For this review, take the finished solid that the model builds, in its own axes (mm). Face numbers are marked on the shaded views. A direction names the side the tool comes from. Round coordinates to 2 decimals unless told otherwise and drop trailing zeros. Write each loop counter-clockwise with the first axis right and the second up, starting at its lowest first coordinate (ties: lowest second). Pieces come first, ordered by that corner, then holes. Notation, with made-up numbers: (67.5, 27.5) - (79.5, 27.5) arc R26 ccw to (79.5, 48.5) - close; hole circle Ø8 at (-11.5, -1). An arc over 180 degrees is marked (long way). One line per item, written item: value. Start each with the question number.
Q1. Add section D-D on z = -15. Write out the cut boundary in (x, y), and give its area (3 significant figures).
Q2. For probe 1 along Z at (x, y) = (-15, 9); probe 2 along X at (y, z) = (9.35, 5); probe 3 along Z at (x, y) = (-15, 1.55), list the stretches that pass through material, from the lowest coordinate up.
Q3. Clearance check with flat-ended pins moving along their axes: pin 1 Ø4 at (y, z) = (19, 5) entering from +X; pin 2 Ø4 at (y, z) = (19.5, 6.5) entering from -X; pin 3 Ø10 at (x, y) = (-26.5, 8) entering from +Z; pin 4 Ø4.5 at (x, z) = (-15, 5) entering from -Y. State where each tip first meets the part, or that it passes through.
Q4. Tool access review of the marked faces 1 and 2: name each direction out of +Z, -Z, +X, -X, +Y, -Y from which nothing blocks a thin tool from reaching the whole face with its end or side.
Q5. Add section A-A on z = 5. Write out the cut boundary in (x, y), and give its area (3 significant figures).
Q6. Add section B-B on x = -15. Write out the cut boundary in (y, z), and give its area (4 significant figures).
Q7. Add section C-C on y = 19.75. Write out the cut boundary in (x, z), and give its area (3 significant figures).
Autodesk Inventor part; units mm, degrees
ref_plane "YZ Plane" through (0, 0, 0) normal (1, 0, 0) x (0, 1, 0)
ref_plane "XZ Plane" through (0, 0, 0) normal (0, 1, 0) x (-1, 0, 0)
ref_plane "XY Plane" through (0, 0, 0) normal (0, 0, 1) x (1, 0, 0)
sketch "Sketch1" plane through (0, 0, 0) normal (0, 1, 0) x (-1, 0, 0)
  line L0 (0, 0) -> (30, 0)
  line L1 (30, 0) -> (30, -80)
  line L2 (30, -80) -> (0, -80)
  line L3 (0, -80) -> (0, 0)
  dimension "d0" = 30
  dimension "d1" = 80
extrude "Extrusion1" add sketch "Sketch1" along normal blind 30
sketch "Sketch2" plane through (-30, 0, 0) normal (0, 0, 1) x (1, 0, 0)
  line L0 (30, 0) -> (0, 0)
  line L1 (15, 0) -> (15, 7.5)
  line L2 (15, 7.5) -> (20, 7.5)
  line L3 (20, 7.5) -> (20, 12.5)
  line L4 (20, 12.5) -> (15, 12.5)
  line L5 (15, 12.5) -> (15, 7.5)
  line L6 (15, 12.5) -> (10, 12.5)
  line L7 (10, 12.5) -> (10, 7.5)
  line L8 (10, 7.5) -> (15, 7.5)
  line L9 (15, 7.5) -> (15, 12.5)
  line L10 (10, 12.5) -> (20, 12.5)
  line L11 (20, 12.5) -> (20, 17.5)
  line L12 (20, 17.5) -> (10, 17.5)
  line L13 (10, 17.5) -> (10, 12.5)
  line L14 (20, 17.5) -> (10, 17.5)
  line L15 (10, 17.5) -> (10, 22.5)
  line L16 (10, 22.5) -> (20, 22.5)
  line L17 (20, 22.5) -> (20, 17.5)
  dimension "d4" = 7.5
  dimension "d5" = 5
  dimension "d6" = 5
  dimension "d7" = 5
  dimension "d8" = 5
  dimension "d9" = 5
  dimension "d10" = 5
extrude "Extrusion2" add sketch "Sketch2" along normal blind 10 contours L5 L4 L3 L2 | L8 L7 L6 L5 | L12 L15 L16 L17
sketch "Sketch3" plane through (-20, 22.5, 0) normal (0, 1, 0) x (1, 0, 0)
  line L0 (0, 0) -> (0, -10)
  line L1 (0, -5) -> (10, -5)
  line L2 (10, 0) -> (10, -10)
  circle A0 centre (5, -5) radius 2.5
  point P0 (20, 0)
  dimension "d13" = 5
extrude "Extrusion3" cut sketch "Sketch3" against normal through all
sketch "Sketch4" plane through (0, 0, 0) normal (0, -1, 0) x (1, 0, 0)
  line L0 (-10, 0) -> (-20, 0)
  line L1 (-15, 0) -> (-15, -15)
  circle A0 centre (-15, -15) radius 2.5
  point P0 (0, 0)
  dimension "d16" = 15
  dimension "d17" = 5
extrude "Extrusion4" cut sketch "Sketch4" against normal blind 5
properties part number "tail"
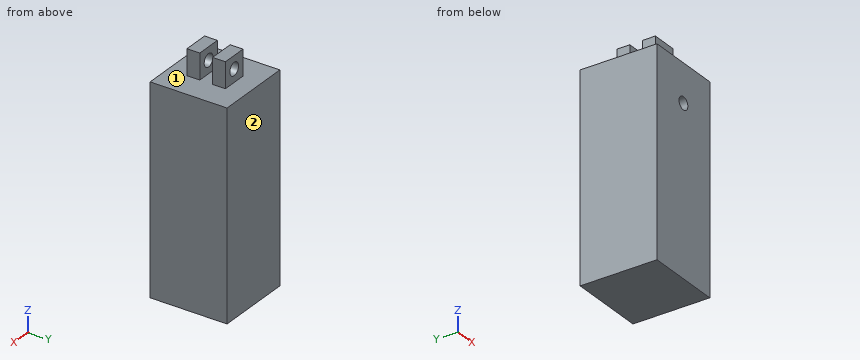
Result set:
1. outline: (-30, 0) - (-17.5, 0) - (-17.5, 5) - (-12.5, 5) - (-12.5, 0) - (0, 0) - (0, 30) - (-30, 30) - close
1. area: 875 mm^2
2. probe 1: z = -80 to 2.5, 7.5 to 10
2. probe 2: x = -20 to -17.5, -12.5 to -10
2. probe 3: z = -80 to -17.5, -12.5 to 0
3. pin 1: stops at x = -10
3. pin 2: stops at x = -20
3. pin 3: stops at z = 0
3. pin 4: passes through
4. face 1: +Z
4. face 2: +Z, -Z, +X, -X, +Y
5. outline: (-20, 7.5) - (-17.5, 7.5) - (-17.5, 12.5) - (-20, 12.5) - close; (-20, 17.5) - (-17.5, 17.5) - (-17.5, 22.5) - (-20, 22.5) - close; (-12.5, 7.5) - (-10, 7.5) - (-10, 12.5) - (-12.5, 12.5) - close; (-12.5, 17.5) - (-10, 17.5) - (-10, 22.5) - (-12.5, 22.5) - close
5. area: 50.0 mm^2
6. outline: (0, -80) - (30, -80) - (30, 0) - (22.5, 0) - (22.5, 2.5) - (17.5, 2.5) - (17.5, 0) - (12.5, 0) - (12.5, 2.5) - (7.5, 2.5) - (7.5, 0) - (0, 0) - (0, -12.5) - (5, -12.5) - (5, -17.5) - (0, -17.5) - close; (7.5, 7.5) - (12.5, 7.5) - (12.5, 10) - (7.5, 10) - close; (17.5, 7.5) - (22.5, 7.5) - (22.5, 10) - (17.5, 10) - close
6. area: 2,425 mm^2
7. outline: (-30, -80) - (0, -80) - (0, 0) - (-10, 0) - (-10, 10) - (-20, 10) - (-20, 0) - (-30, 0) - close; hole circle Ø5 at (-15, 5)
7. area: 2,480 mm^2
